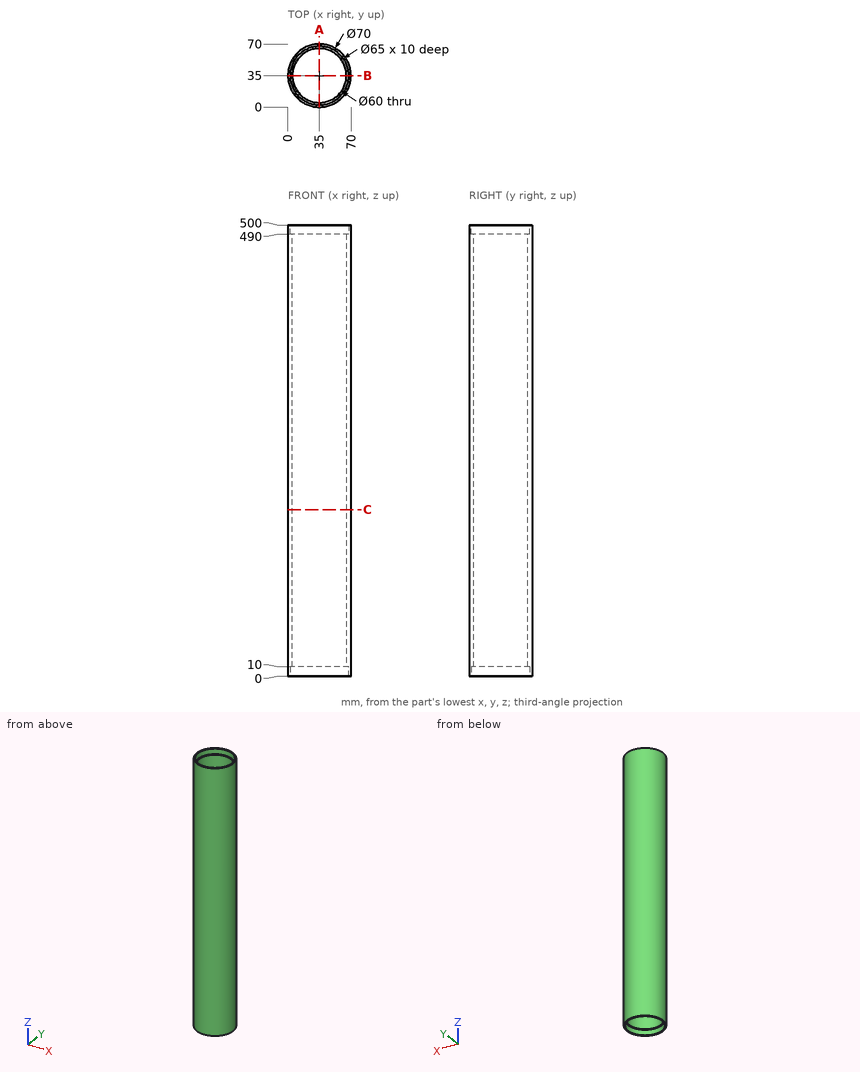
The figure shows three views and two pictorial views of one solid part (mm, origin at its lowest corner). Answer the questions. Coordinates: 2 decimals unless noted, no trailing zeros. Loops run counter-clockwise (first coordinate to the right, second up) from the corner with the lowest first, then second, coordinate; pieces in that order, holes last. Notation, with made-up numbers: (45.25, 17.25) -> (49.25, 17.25) arc R35 ccw to (49.25, 51.25) -> close; hole circle Ø7 at (37, 85). An arc over 180 degrees is marked (long way). Write item = value, one per line. Start each with the question number.
1) Given pin 1 Ø12 at (x, z) = (51.5, 388.5) entering from +Y; pin 2 Ø1 at (y, z) = (19.5, 58) entering from -X; pin 3 Ø2 at (x, z) = (30.5, 394.5) entering from -Y, each flat-ended and moving along its own axis, determine where each tip first touches the part or whether it passes through.
2) Straight lines are drawn through the part: line 1 (Y direction, x = 35, z = 2.5); line 2 (X direction, y = 33.5, z = 289.5); line 3 (X direction, y = 37.5, z = 175). For each, find the intervals that lie inside material, in ascending order. Write a range as from..to.
3) A cutting plane is placed at C-C (z = 184.5). Give the vertices of the cut face in (x, y), then the cut area to 3 significant figures.
4) A cutting plane is placed at A-A (x = 35). Give the vertices of the cut face in (y, z).
Responses:
q1.pin_1 = 68.39
q1.pin_2 = 3.38
q1.pin_3 = 0.18
q2.line_1 = 0..2.5, 67.5..70
q2.line_2 = 0.03..5.04, 64.96..69.97
q2.line_3 = 0.09..5.1, 64.9..69.91
q3.outline = circle Ø70 at (35, 35); hole circle Ø60 at (35, 35)
q3.area = 1,020 mm²
q4.outline = (0, 0) -> (2.5, 0) -> (2.5, 10) -> (5, 10) -> (5, 490) -> (2.5, 490) -> (2.5, 500) -> (0, 500) -> close; (65, 10) -> (67.5, 10) -> (67.5, 0) -> (70, 0) -> (70, 500) -> (67.5, 500) -> (67.5, 490) -> (65, 490) -> close
